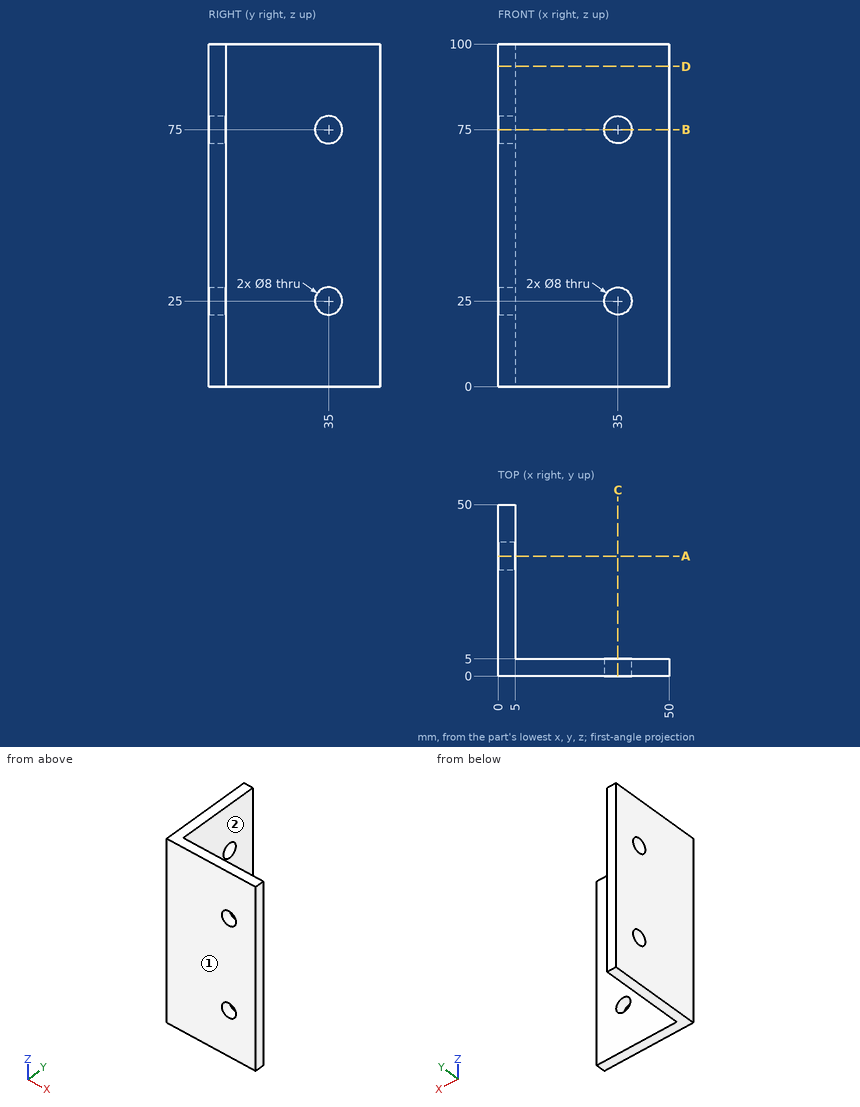
Here's the drawing with two shaded views (mm, measured from the low corner). I have some questions. A direction names the side the tool comes from. Coordinates: 2 decimals unless noted, no trailing zeros. Write each loop counter-clockwise with the first axis right and the second up, starting at its lowest first coordinate (ties: lowest second). Pieces come first, ordered by that corner, then holes. Notation, with made-up numbers: (58.25, 80) -> (76.25, 80) arc R36 cw to (76.25, 114) -> close; hole circle Ø5 at (-1.75, 44.5). An arc over 180 degrees is marked (long way). Use a Markdown table: item, result. Add a question column.
(1) I'm going to push flat-ended pins straight in: P1, Ø8, axis at x = 45, y = 12, coming from the -Z side; P2, Ø1.5, axis at y = 19.5, z = 76, coming from the +X side; P3, Ø22.5, axis at x = 28, z = 42.5, coming from the +Y side. Where does each tip first touch, or does it pass through?
(2) For the marked faces 1 and 2, which set-ups out of +Z, -Z, +X, -X, +Y, -Y let a thin tool reach every point of the face, with its end or its side?
(3) Please list where these lines run through material, in increasing order: line 1 (Z direction, x = 1, y = 35); line 2 (Y direction, x = 27, z = 59).
(4) If we section it at A-A, the plane y = 35: Write out the boundary of the cut face in (x, z).
(5) If we section it at B-B, the plane z = 75: Write out the boundary of the cut face in (x, y).
(6) If we section it at D-D, the plane z = 93.5: Write out the boundary of the cut face in (x, y).
Outcome:
| question | item | result |
|---|---|---|
| 1 | P1 | passes through |
| 1 | P2 | stops at x = 5 |
| 1 | P3 | stops at y = 5 |
| 2 | face 1 | +Z, -Z, +X, -X, -Y |
| 2 | face 2 | +Z, -Z, +X, +Y |
| 3 | line 1 | z = 0 to 21, 29 to 71, 79 to 100 |
| 3 | line 2 | y = 0 to 5 |
| 4 | outline | (0, 0) -> (5, 0) -> (5, 21) -> (0, 21) -> close; (0, 29) -> (5, 29) -> (5, 71) -> (0, 71) -> close; (0, 79) -> (5, 79) -> (5, 100) -> (0, 100) -> close |
| 5 | outline | (0, 0) -> (31, 0) -> (31, 5) -> (5, 5) -> (5, 31) -> (0, 31) -> close; (0, 39) -> (5, 39) -> (5, 50) -> (0, 50) -> close; (39, 0) -> (50, 0) -> (50, 5) -> (39, 5) -> close |
| 6 | outline | (0, 0) -> (50, 0) -> (50, 5) -> (5, 5) -> (5, 50) -> (0, 50) -> close |
